Print and shaded views of the part. All mm, measured from the part's lowest x, y and z. A direction names the side the tool comes from. Round coordinates to 2 decimals unless told otherwise and drop trailing zeros. Write each loop counter-clockwise with the first axis right and the second up, starting at its lowest first coordinate (ties: lowest second). Pieces come first, ordered by that corner, then holes. Notation, with made-up numbers: (80.25, -14.5) - (105.25, -14.5) arc R34 cw to (105.25, 18.5) - close; hole circle Ø10 at (28.25, 18). An arc over 180 degrees is marked (long way). One line per item, written item: value.
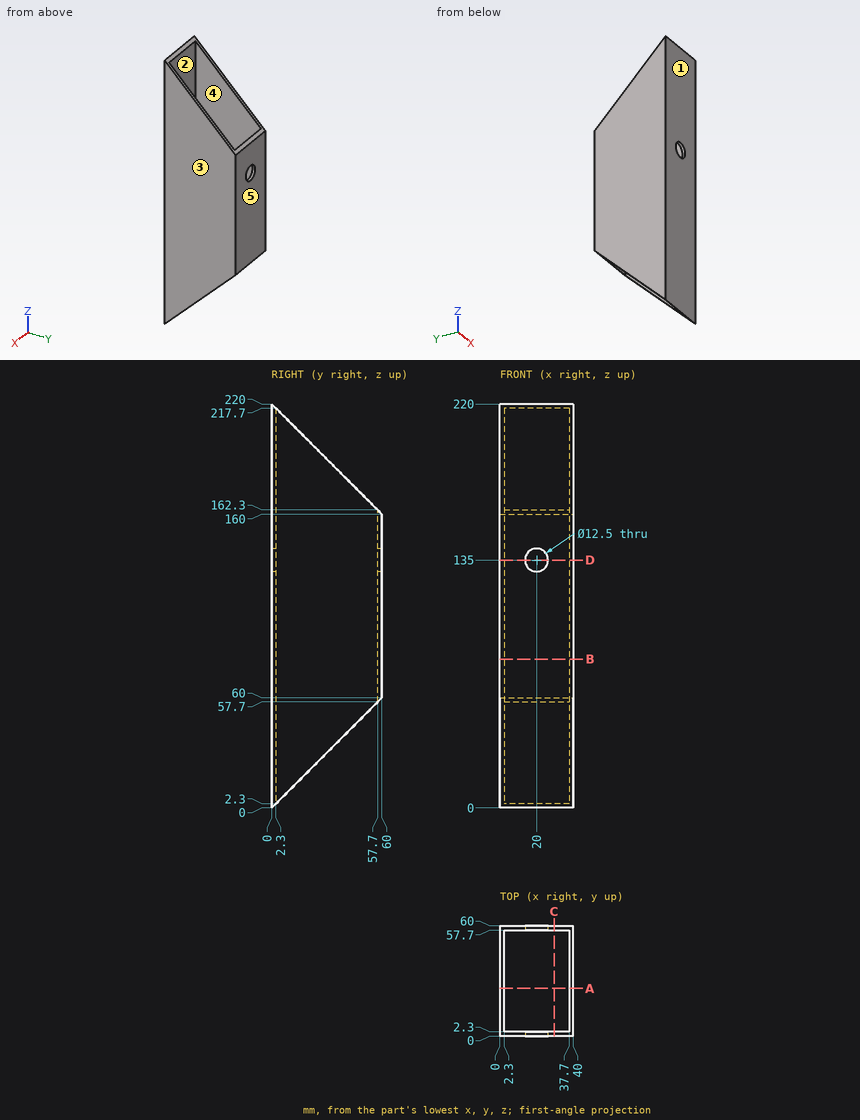
1. Wall check: probe 1 along X at (y, z) = (14, 97.5); probe 2 along Y at (x, z) = (20, 67); probe 3 along Z at (x, y) = (20, 58.95). Give the ranges that are in metal, low to high. Write a range as [from, to].
Report:
probe 1: [0, 2.3], [37.7, 40]
probe 2: [0, 2.3], [57.7, 60]
probe 3: [58.95, 128.75], [141.25, 161.05]
2. Band-saw the part on D-D on z = 135. Write the cut outline in (x, y), plus the area to 3 significant figures.
Report:
outline: (0, 0) - (13.75, 0) - (13.75, 2.3) - (2.3, 2.3) - (2.3, 57.7) - (13.75, 57.7) - (13.75, 60) - (0, 60) - close; (26.25, 0) - (40, 0) - (40, 60) - (26.25, 60) - (26.25, 57.7) - (37.7, 57.7) - (37.7, 2.3) - (26.25, 2.3) - close
area: 381 mm²
3. Band-saw the part on B-B on z = 81. Write the cut outline in (x, y).
Report:
outline: (0, 0) - (40, 0) - (40, 60) - (0, 60) - close; hole (2.3, 2.3) - (37.7, 2.3) - (37.7, 57.7) - (2.3, 57.7) - close
4. Tool access for the marked faces 4 and 5: list every direction of +Z, -Z, +X, -X, +Y, -Y with a clear straight run to the whole face (end or side of a thin tool).
Report:
face 4: +Z, -Z
face 5: +Z, -Z, +X, -X, +Y
5. Mould opens along Y. For the marked faces 1, 2 and 3 say: released by +Y, released by -Y, zero draft, split by the parting line, or undercut.
Report:
face 1: released by -Y
face 2: undercut
face 3: zero draft
6. Drop a flat-ended pin along its axis: pin 1 (7.5 mm diameter, centred on x = 20, z = 135, fed in from +Y). Give the stop position or say it passes through.
Report:
pin 1: through
7. Band-saw the part on A-A on y = 26. Write the cut outline in (x, z), plus the area to 3 significant figures.
Report:
outline: (0, 26) - (2.3, 26) - (2.3, 194) - (0, 194) - close; (37.7, 26) - (40, 26) - (40, 194) - (37.7, 194) - close
area: 773 mm²
8. Band-saw the part on C-C on x = 29.5. Write the cut outline in (y, z), plus the area to 3 significant figures.
Report:
outline: (0, 0) - (2.3, 2.3) - (2.3, 217.7) - (0, 220) - close; (57.7, 57.7) - (60, 60) - (60, 160) - (57.7, 162.3) - close
area: 736 mm²
